```python
from build123d import *

# Parameters (mm, degrees)
SKETCH1_R                   = 11.1125
BOSS_EXTRUDE1_DEPTH         = 9.525
BOSS_EXTRUDE1_DEPTH_BACK    = 9.525
SKETCH2_R                   = 6.35
BOSS_EXTRUDE2_DEPTH         = 101.6
F_1_2_CLEARANCE_HOLE1_D     = 13.49248
F_1_2_CLEARANCE_HOLE1_DEPTH = 63.5
F_1_2_CLEARANCE_HOLE1_TIP   = 4.053549943


with BuildPart() as part:
    # Sketch1 → Boss-Extrude1 (new body, two sides)
    with BuildSketch(Plane.XY) as boss_extrude1_sk:
        Circle(SKETCH1_R)
    extrude(amount=BOSS_EXTRUDE1_DEPTH)
    extrude(boss_extrude1_sk.sketch, amount=-BOSS_EXTRUDE1_DEPTH_BACK)

    # Sketch2 → Boss-Extrude2 (add)
    with BuildSketch(Plane(origin=(0, 0, 0), x_dir=(1, 0, 0), z_dir=(0, 1, 0))):
        Circle(SKETCH2_R)
    extrude(amount=BOSS_EXTRUDE2_DEPTH)

    # 1_2 Clearance Hole1
    with Locations(Plane.XY.offset(9.525)):
        with Locations((0, 0)):
            Hole(F_1_2_CLEARANCE_HOLE1_D / 2, depth=F_1_2_CLEARANCE_HOLE1_DEPTH)
            with Locations((0, 0, -(F_1_2_CLEARANCE_HOLE1_DEPTH + F_1_2_CLEARANCE_HOLE1_TIP / 2))):  # 118° drill point
                Cone(0, F_1_2_CLEARANCE_HOLE1_D / 2, F_1_2_CLEARANCE_HOLE1_TIP, mode=Mode.SUBTRACT)


solid = part.part
```
Work out the finished part from the listing and answer in its coordinate system (mm). Round coordinates to 2 decimals unless told otherwise and drop trailing zeros. Write each loop counter-clockwise with the first axis right and the second up, starting at its lowest first coordinate (ties: lowest second). Pieces come first, ordered by that corner, then holes. Notation, with made-up numbers: (88, -17.75) -> (144, -17.75) arc R15 ccw to (144, 5.25) -> close; hole circle Ø9 at (15.5, 30). An arc over 180 degrees is marked (long way). Write each question's results on one line, items separated by ' | '.
1) Flat-ended cylindrical pins translate along their axes: pin 1 (6 mm diameter, centred on y = 73.5, z = 7, fed in from +X); pin 2 (8 mm diameter, centred on x = 0, z = 7.5, fed in from +Y); pin 3 (6 mm diameter, centred on y = 39.5, z = 2.5, fed in from -X); pin 4 (12 mm diameter, centred on x = 5.5, y = 73, fed in from +Z). Find the tip coordinate at first contact, or state that the pin passes through.
Findings:
pin 1: stops at x = 4.93 | pin 2: stops at y = 101.6 | pin 3: stops at x = -6.35 | pin 4: stops at z = 6.35
2) The part is cut by section D-D (x = 5.25). Write down the section's boundary in (y, z) (3 decimals), and give its area (3 significant figures).
Findings:
outline: (-9.794, -9.525) -> (-4.237, -9.525) -> (-4.237, 9.525) -> (-9.794, 9.525) -> close; (4.237, -9.525) -> (9.794, -9.525) -> (9.794, -3.572) -> (101.6, -3.572) -> (101.6, 3.572) -> (9.794, 3.572) -> (9.794, 9.525) -> (4.237, 9.525) -> close | area: 868 mm²
3) The part is cut by section B-B (y = 0). Write down the section's boundary in (x, z) (1 decimal).
Findings:
outline: (-11.1, -9.5) -> (-6.7, -9.5) -> (-6.7, 9.5) -> (-11.1, 9.5) -> close; (6.7, -9.5) -> (11.1, -9.5) -> (11.1, 9.5) -> (6.7, 9.5) -> close
4) Consider line 1 along X through (y, z) = (-0.5, -6.5); line 2 along Y through (x, z) = (0, -0.5); line 3 along Y through (x, z) = (3.5, -8). Determine where each line is inside the solid, lowest interval first. Write a range as [from, to].
Findings:
line 1: x = [-11.1, -6.73], [6.73, 11.1] | line 2: y = [-11.11, -6.75], [6.75, 101.6] | line 3: y = [-10.55, -5.77], [5.77, 10.55]
5) For a pull along X with two mould halves and no side action, classify faces 1 (the cylindrical face through (-6.435, 2.026, -0.133)), 2 (the flat face through (5, -5, -9.525)), 3 (the cylindrical face through (-1.38, 54.71, 6.2)) as +X half, -X half, draft (parallel to the pull), parting line (faces both ways), or undercut.
Findings:
face 1: undercut | face 2: draft | face 3: parting line
